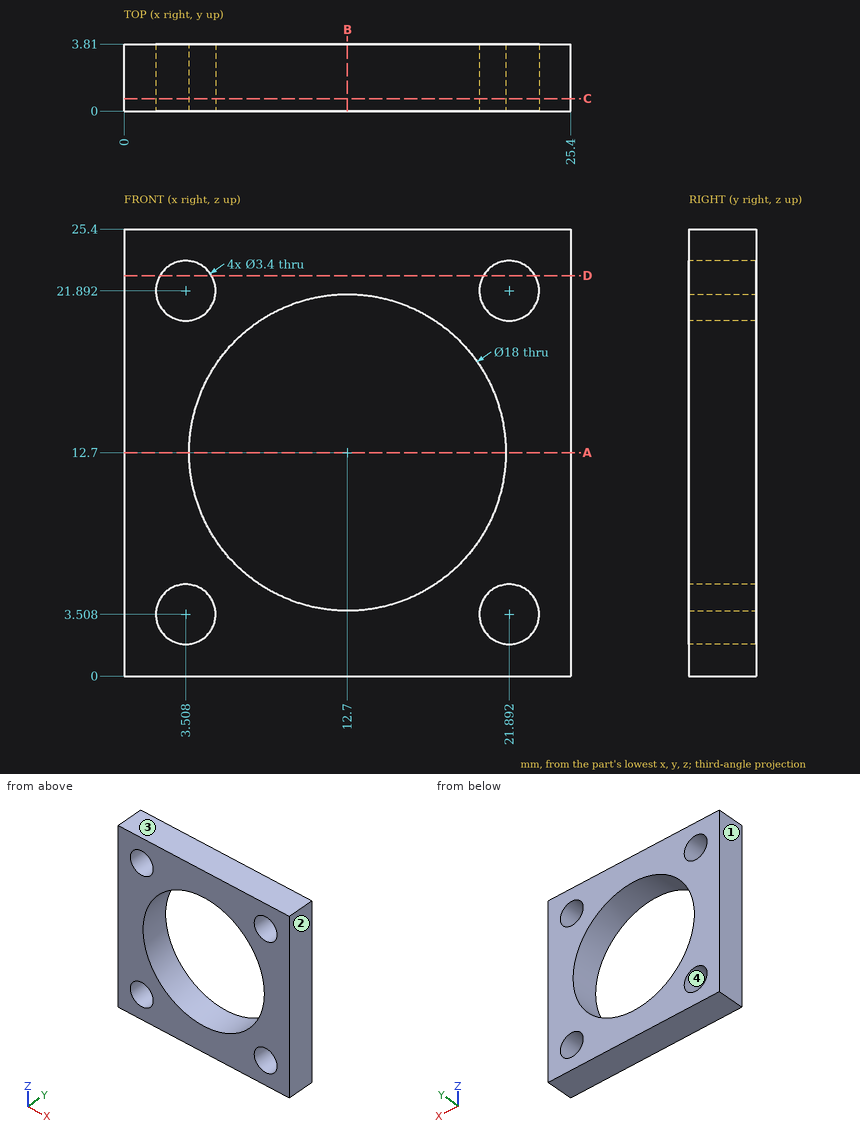
Drawing for the job (mm, zero at the part's lowest x, y, z). Give positions to 0.01 mm unless a question says otherwise; leave off trailing zeros. Order: outer loops, then holes, each group sorted by start corner. A loop starts at its lowest first (then second) coordinate and runs counter-clockwise, first axis right, second up. Notation, with made-up numbers: (-23, 0.25) - (17, 0.25) arc R36 cw to (17, 37.25) - close; hole circle Ø4 at (-28, 70.25). An arc over 180 degrees is marked (long way). Write item = value, one per line. Start each with the question number.
1. Cut at D-D, the plane z = 22.75. List the corners of the cut face in (x, y) (1 decimal).
2. Drop flat-ended pins along their axis: P1, Ø4.5, axis at x = 3.51, z = 3.51, coming from the -Y side; P2, Ø1, axis at x = 17, z = 19, coming from the +Y side. Give the stop position or say it passes through.
3. Cut at C-C, the plane y = 0.7. List the corners of the cut face in (x, z).
4. Cut at B-B, the plane x = 12.7. List the corners of the cut face in (y, z), and give its area (3 significant figures).
5. Two-plate mould, pull along X, no slides. Class the marked faces 1, 2, 3 and 4: pulls with the +X half, pulls with the -X half, needs draft (parallel to the pull), parting line crosses it, or undercut.
6. Probe line 1 along Z through (x, y) = (13, 0.85) (1 decimal); line 2 along X through (y, z) = (1.15, 22) (1 decimal). List the from-to ranges inside material, lowest first.
7. Cut at A-A, the plane z = 12.7. List the corners of the cut face in (x, y).
Taken from the geometry:
q1.outline = (0, 0) - (2, 0) - (2, 3.8) - (0, 3.8) - close; (5, 0) - (20.4, 0) - (20.4, 3.8) - (5, 3.8) - close; (23.4, 0) - (25.4, 0) - (25.4, 3.8) - (23.4, 3.8) - close
q2.P1 = 0
q2.P2 = through
q3.outline = (0, 0) - (25.4, 0) - (25.4, 25.4) - (0, 25.4) - close; hole circle Ø3.4 at (3.51, 3.51); hole circle Ø3.4 at (3.51, 21.89); hole circle Ø18 at (12.7, 12.7); hole circle Ø3.4 at (21.89, 3.51); hole circle Ø3.4 at (21.89, 21.89)
q4.outline = (0, 0) - (3.81, 0) - (3.81, 3.7) - (0, 3.7) - close; (0, 21.7) - (3.81, 21.7) - (3.81, 25.4) - (0, 25.4) - close
q4.area = 28.2 mm²
q5.face_1 = pulls with the -X half
q5.face_2 = pulls with the +X half
q5.face_3 = needs draft
q5.face_4 = undercut
q6.line_1 = 0 to 3.7, 21.7 to 25.4
q6.line_2 = 0 to 1.8, 5.2 to 20.2, 23.6 to 25.4
q7.outline = (0, 0) - (3.7, 0) - (3.7, 3.81) - (0, 3.81) - close; (21.7, 0) - (25.4, 0) - (25.4, 3.81) - (21.7, 3.81) - close
